```python
from build123d import *

# Parameters (mm, degrees)
F0_W     = 29.94
F0_H     = 25.4
F1_DEPTH = 11.3
F2_W     = 11.3
F2_H     = 11.3
F3_DEPTH = 25
F4_R     = 2
F5_R     = 1


with BuildPart() as f1:
    # F0 (on Top) → F1 (new body)
    with BuildSketch(Plane.XY):
        with Locations((14.97, 12.7)):
            Rectangle(F0_W, F0_H)
    extrude(amount=F1_DEPTH)

    # F2 (on face) → F3 (cut)
    with BuildSketch(Plane.XY.offset(11.3)):
        with Locations((5.65, 5.65)):
            Rectangle(F2_W, F2_H)
    extrude(amount=-F3_DEPTH, mode=Mode.SUBTRACT)

    # F4
    f4_edges = [f1.edges().sort_by_distance(p)[0] for p in [
        (20.62, 0, 0),
        (0, 18.35, 0),
    ]]
    fillet(f4_edges, radius=F4_R)

    # F5
    f5_edges = [f1.edges().sort_by_distance(p)[0] for p in [
        (29.94, 25.4, 5.65),
        (14.97, 25.4, 11.3),
        (29.94, 12.7, 11.3),
    ]]
    fillet(f5_edges, radius=F5_R)


solid = f1.part
```
The listing builds one solid part. Answer for the finished solid, in the listing's coordinates (mm). A direction names the side the tool comes from. Coordinates: 2 decimals unless noted, no trailing zeros. Loops run counter-clockwise (first coordinate to the right, second up) from the corner with the lowest first, then second, coordinate; pieces in that order, holes last. Notation, with made-up numbers: (12.5, 39.25) -> (60.5, 39.25) arc R7 cw to (60.5, 43.25) -> close; hole circle Ø1 at (69.5, -26). An arc over 180 degrees is marked (long way). Use one line per item in the form item = value. Start each with the question number.
Item 1: The part is cut by section A-A on z = 5.5. Determine the outline of the cut face in (x, y).
Item 2: A tool of negligible diameter and unlimited length cuts with its end or side. For faces 1 (the face through (6, 11.3, 6)), 2 (the face through (29.639, 25.115, 5.222)), from which of +Z, -Z, +X, -X, +Y, -Y can it reach the whole face along a straight path? Write none if from no direction.
Item 3: The part is cut by section B-B on y = 10. Determine the outline of the cut face in (x, z).
Item 4: The part is cut by section C-C on x = 3.5. Determine the outline of the cut face in (y, z), then the cut area to 3 significant figures.
Item 5: Consider L1, parallel to X at y = 3, z = 5.5; L2, parallel to Y at x = 4.5, z = 6.75; L3, parallel to Y at x = 28.5, z = 1.25. Determine where each line is inside the solid, lowest interval first. Write a range as [from, to].
Answer key:
q1.outline = (0, 11.3) -> (11.3, 11.3) -> (11.3, 0) -> (29.94, 0) -> (29.94, 24.4) arc R1 ccw to (28.94, 25.4) -> (0, 25.4) -> close
q2.face_1 = +Z, -Z, -X, -Y
q2.face_2 = +Z, -Z, +X, +Y
q3.outline = (11.3, 0) -> (29.94, 0) -> (29.94, 10.3) arc R1 ccw to (28.94, 11.3) -> (11.3, 11.3) -> close
q4.outline = (11.3, 0) -> (25.4, 0) -> (25.4, 10.3) arc R1 ccw to (24.4, 11.3) -> (11.3, 11.3) -> close
q4.area = 159 mm2
q5.L1 = [11.3, 29.94]
q5.L2 = [11.3, 25.4]
q5.L3 = [0.15, 25.4]
